Build history of the part. All positions in model axes, mm. Give positions to 0.01 mm unless a question says otherwise; leave off trailing zeros. Write each loop counter-clockwise with the first axis right and the second up, starting at its lowest first coordinate (ties: lowest second). Pieces come first, ordered by that corner, then holes. Notation, with made-up numbers: (-24.75, 17.25) -> (-15.75, 17.25) arc R24 ccw to (-15.75, 37.25) -> close; hole circle Ø8 at (16, -7.75). An arc over 180 degrees is marked (long way). Put each result on its own line as item: value.
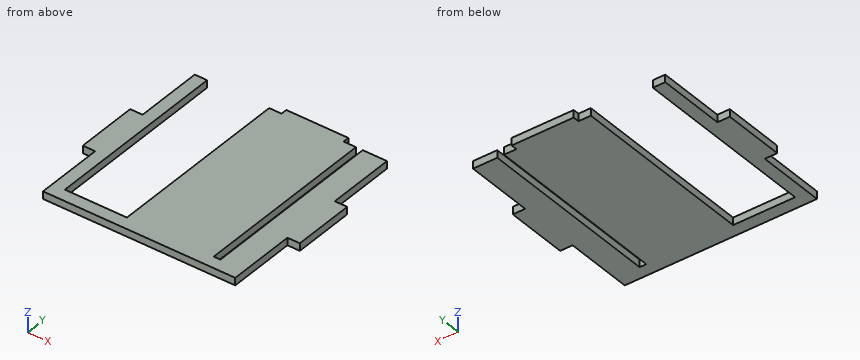
from build123d import *

# Parameters (mm, degrees)
SKETCH1_W           = 10
SKETCH1_H           = 50
SKETCH1_W_2         = 50
SKETCH1_H_2         = 5
BOSS_EXTRUDE1_DEPTH = 6


with BuildPart() as part:
    # Sketch1 → Boss-Extrude1 (new body)
    with BuildSketch(Plane.XY):
        Polygon((-155, 0), (0, 0), (0, 55), (0, 105), (0, 160), (-19.6, 160), (-19.6, 10), (-25, 10), (-25, 160), (-35, 160), (-72.61115591, 160), (-77.64696312, 160), (-85, 160), (-95, 160), (-95, 10), (-145, 10), (-145, 160), (-155, 160), (-155, 105), (-155, 55), align=None)
        with Locations((-160, 80)):
            Rectangle(SKETCH1_W, SKETCH1_H)
        with Locations((5, 80)):
            Rectangle(SKETCH1_W, SKETCH1_H)
        with Locations((-60, 162.5)):
            Rectangle(SKETCH1_W_2, SKETCH1_H_2)
    extrude(amount=BOSS_EXTRUDE1_DEPTH)


solid = part.part
1) Wall check: L1, parallel to X at y = 39, z = 1.5; L2, parallel to X at y = 67, z = 3.3; L3, parallel to Y at x = -156, z = 2.75. Give the ranges that are in metal, low to high.
Filled sheet:
L1: -155 to -145, -95 to -25, -19.6 to 0
L2: -165 to -145, -95 to -25, -19.6 to 10
L3: 55 to 105
2) Pin check, flat tips, straight feed: pin 1 (1.5 mm diameter, centred on y = 162.5, z = 2, fed in from +X); pin 2 (1.8 mm diameter, centred on x = -122.5, z = 1.5, fed in from +Y); pin 3 (3 mm diameter, centred on x = -149, z = 4.5, fed in from +Y). Stop position of each tip, or through.
Filled sheet:
pin 1: x = -35
pin 2: y = 10
pin 3: y = 160
3) Slice it at C-C (y = 138.5). Write the cut outline in (x, z), plus the area to 3 significant figures.
Filled sheet:
outline: (-155, 0) -> (-145, 0) -> (-145, 6) -> (-155, 6) -> close; (-95, 0) -> (-25, 0) -> (-25, 6) -> (-95, 6) -> close; (-19.6, 0) -> (0, 0) -> (0, 6) -> (-19.6, 6) -> close
area: 598 mm2
4) Slice it at A-A (y = 69). Write the cut outline in (x, z), plus the area to 3 significant figures.
Filled sheet:
outline: (-165, 0) -> (-145, 0) -> (-145, 6) -> (-165, 6) -> close; (-95, 0) -> (-25, 0) -> (-25, 6) -> (-95, 6) -> close; (-19.6, 0) -> (10, 0) -> (10, 6) -> (-19.6, 6) -> close
area: 718 mm2
5) Slice it at B-B (z = 3.95). Write the cut outline in (x, y).
Filled sheet:
outline: (-165, 55) -> (-155, 55) -> (-155, 0) -> (0, 0) -> (0, 55) -> (10, 55) -> (10, 105) -> (0, 105) -> (0, 160) -> (-19.6, 160) -> (-19.6, 10) -> (-25, 10) -> (-25, 160) -> (-35, 160) -> (-35, 165) -> (-85, 165) -> (-85, 160) -> (-95, 160) -> (-95, 10) -> (-145, 10) -> (-145, 160) -> (-155, 160) -> (-155, 105) -> (-165, 105) -> close
6) Slice it at D-D (x = -5.5). Write the cut outline in (y, z), plus the area to 3 significant figures.
Filled sheet:
outline: (0, 0) -> (160, 0) -> (160, 6) -> (0, 6) -> close
area: 960 mm2
